The listing builds one solid part. Answer for the finished solid, in the listing's coordinates (mm). Coordinates: 2 decimals unless noted, no trailing zeros. Loops run counter-clockwise (first coordinate to the right, second up) from the corner with the lowest first, then second, coordinate; pieces in that order, holes last. Notation, with made-up numbers: M -34.5,-11 L 18.5,-11 A20 cw 18.5,0 Z; hole C -9,68.25 d9. An arc over 180 degrees is marked long. Answer as a JSON object with one key per item and string values. Group by question number.
1. Straight lines are drawn through the part: L1, parallel to Z at x = 36, y = -18; L2, parallel to X at y = -7.75, z = -16; L3, parallel to X at y = -16.25, z = -14.5. For each, find the intervals that lie inside material, in ascending order.
2. Given pin 1 (1.5 mm diameter, centred on x = 36, y = -6.5, fed in from +Z); pin 2 (1.5 mm diameter, centred on y = -2.5, z = -7, fed in from -X); pin 3 (3 mm diameter, centred on y = -6.5, z = -18, fed in from +X); pin 4 (6 mm diameter, centred on x = 7.5, y = -3, fed in from -Z), each flat-ended and moving along its own axis, determine where each tip first touches the part or whether it passes through.
3. Determine the mould class of faces 1 (the face through (33.464, -9.705, -15.597)), 2 (the face through (0, -10, -3)), 3 (the face through (36.724, -9.705, -22.163)) for opening direction Z: released by +Z, released by -Z, zero draft, split by the parting line, or undercut.
4. A cutting plane is placed at C-C on x = 35. Give the vertices of the cut face in (y, z) (3 decimals), and give its area (3 significant figures).
5. A cutting plane is placed at A-A on z = -14. Give the vertices of the cut face in (x, y) (3 decimals).
6. A cutting plane is placed at D-D on z = -9.5. Give the vertices of the cut face in (x, y) (3 decimals), and give its area (3 significant figures).
7. A cutting plane is placed at B-B on y = -15. Give the vertices of the cut face in (x, z), and give its area (3 significant figures).
from build123d import *

# Parameters (mm, degrees)
SKETCH1_R           = 2.38125
BOSS_EXTRUDE1_DEPTH = 19.685


with BuildPart() as part:
    # Sketch1 → Boss-Extrude1 (new body)
    with BuildSketch(Plane(origin=(0, 0, 0), x_dir=(1, 0, 0), z_dir=(0, 1, 0))):
        with BuildLine():
            Line((0, 5.08), (32.579112959, 21.463440611))
            ThreePointArc((32.579112959, 21.463440611), (36.78416415, 22.155288174), (40.634925166, 20.329706577))
            Line((40.634925166, 20.329706577), (57.15, 5.08))
            Line((57.15, 5.08), (57.15, 0))
            Line((57.15, 0), (0, 0))
            Line((0, 0), (0, 5.08))
        make_face()
        with Locations(Location((35.7886, 15.08125, 0), (0, 0, 270))):
            Circle(SKETCH1_R, mode=Mode.SUBTRACT)
    extrude(amount=-BOSS_EXTRUDE1_DEPTH)


solid = part.part
From the geometry:
{
 "1": {"L1": "z = -22.22 to -17.45, -12.71 to 0", "L2": "x = 21.71 to 33.59, 37.99 to 45.32", "L3": "x = 18.73 to 33.48, 38.1 to 46.95"},
 "2": {"pin 1": "stops at z = 0", "pin 2": "stops at x = 2.33", "pin 3": "stops at x = 44.78", "pin 4": "stops at z = -10.36"},
 "3": {"face 1": "undercut", "face 2": "zero draft", "face 3": "released by -Z"},
 "4": {"outline": "M -19.685,-22.181 L 0,-22.181 L 0,-17.328 L -19.685,-17.328 Z; M -19.685,-12.834 L 0,-12.834 L 0,0 L -19.685,0 Z", "area": "348 mm²"},
 "5": {"outline": "M 17.738,-19.685 L 33.667,-19.685 L 33.667,0 L 17.738,0 Z; M 37.91,-19.685 L 47.49,-19.685 L 47.49,0 L 37.91,0 Z"},
 "6": {"outline": "M 8.789,-19.685 L 52.363,-19.685 L 52.363,0 L 8.789,0 Z", "area": "858 mm²"},
 "7": {"outline": "M 0,-5.08 L 32.58,-21.46 A7.14 ccw 40.63,-20.33 L 57.15,-5.08 L 57.15,0 L 0,0 Z; hole C 35.79,-15.08 d4.76", "area": "800 mm²"}
}
